Input: part model. Units: mm. Frame: model coordinates. A direction names the side the tool comes from. Give positions to 0.01 mm unless a question says otherwise; leave off trailing zeros. Loops run counter-clockwise (first coordinate to the right, second up) from the corner with the lowest first, then second, coordinate; pieces in that order, holes last. Notation, with made-up numbers: (-30, 35) -> (1, 35) arc R10 cw to (1, 39) -> close; hole circle Ø5 at (38.5, 81.5). An arc over 180 degrees is marked (long way). Answer as a JSON object with one key per item and string values. Group by question number.
Autodesk Inventor part; units mm, degrees
ref_plane "YZ Plane" through (0, 0, 0) normal (1, 0, 0) x (0, 1, 0)
ref_plane "XZ Plane" through (0, 0, 0) normal (0, 1, 0) x (-1, 0, 0)
ref_plane "XY Plane" through (0, 0, 0) normal (0, 0, 1) x (1, 0, 0)
sketch "Sketch2" plane through (0, 0, 0) normal (0, 0, 1) x (1, 0, 0)
  line L0 (0, 12.7) -> (3.6703, 12.7)
  line L1 (0, 12.7) -> (-3.6703, 12.7)
  line L2 (0, 0) -> (3.6703, 0)
  line L3 (0, 0) -> (-3.6703, 0)
  line L4 (-3.6703, 0) -> (-7.3406, 6.35)
  line L5 (-7.3406, 6.35) -> (-3.6703, 12.7)
  line L6 (3.6703, 12.7) -> (7.3406, 6.35)
  line L7 (7.3406, 6.35) -> (3.6703, 0)
  line L8 (0, 0) -> (0, 6.35)
  circle A0 centre (0, 6.35) radius 8.255
  dimension "d11" = 6.35
  dimension "d12" = 16.51
extrude "Extrusion2" add sketch "Sketch2" along normal blind 6.223
sketch "Sketch3" plane through (0, 6.35, 6.223) normal (0, 0, 1) x (1, 0, 0)
  line L0 (-3.6703, -6.35) -> (-7.3406, 0)
  line L1 (-7.3406, 0) -> (-3.6703, 6.35)
  line L2 (-3.6703, 6.35) -> (3.6703, 6.35)
  line L3 (3.6703, 6.35) -> (7.3406, 0)
  line L4 (7.3406, 0) -> (3.6703, -6.35)
  line L5 (3.6703, -6.35) -> (-3.6703, -6.35)
  circle A0 centre (0, 0) radius 8.255
  point P0 (0, -6.35)
extrude "Extrusion3" add sketch "Sketch3" along normal blind 3.302
sketch "Sketch4" plane through (0, 6.35, 9.525) normal (0, 0, 1) x (1, 0, 0)
  line L0 (-7.3406, 0) -> (-3.6703, 6.35)
  line L1 (-3.6703, 6.35) -> (3.6703, 6.35)
  line L2 (3.6703, 6.35) -> (7.3406, 0)
  line L3 (7.3406, 0) -> (3.6703, -6.35)
  line L4 (3.6703, -6.35) -> (-3.6703, -6.35)
  line L5 (-3.6703, -6.35) -> (-7.3406, 0)
  circle A0 centre (0, 0) radius 8.255
  point P0 (0, -6.35)
extrude "Extrusion4" add sketch "Sketch4" along normal blind 6.5786
sketch "Sketch5" plane through (0, 6.35, 16.1036) normal (0, 0, 1) x (1, 0, 0)
  line L0 (-16.3467, 15.7745) -> (15.1254, 15.7745)
  line L1 (15.1254, 15.7745) -> (15.1254, -12.8793)
  line L2 (15.1254, -12.8793) -> (-16.3467, -12.8793)
  line L3 (-16.3467, -12.8793) -> (-16.3467, 15.7745)
  point P0 (0, -6.35)
extrude "Extrusion5" cut sketch "Sketch5" against normal blind 6.5786
sketch "Sketch8" plane through (0, 6.35, 9.525) normal (0, 0, 1) x (1, 0, 0)
  line L0 (-7.3406, 0) -> (-3.6703, -6.35)
  line L1 (-3.6703, 6.35) -> (-7.3406, 0)
  line L2 (3.6703, 6.35) -> (-3.6703, 6.35)
  line L3 (7.3406, 0) -> (3.6703, 6.35)
  line L4 (3.6703, -6.35) -> (7.3406, 0)
  line L5 (-3.6703, -6.35) -> (3.6703, -6.35)
  circle A0 centre (0, 0) radius 8.255
  point P0 (0, -6.35)
extrude "Extrusion7" add sketch "Sketch8" along normal blind 15.875
sketch "Sketch9" plane through (0, 6.35, 25.4) normal (0, 0, 1) x (1, 0, 0)
  line L0 (-7.3406, 0) -> (-3.6703, 6.35)
  line L1 (-3.6703, 6.35) -> (3.6703, 6.35)
  line L2 (3.6703, 6.35) -> (7.3406, 0)
  line L3 (7.3406, 0) -> (3.6703, -6.35)
  line L4 (3.6703, -6.35) -> (-3.6703, -6.35)
  line L5 (-3.6703, -6.35) -> (-7.3406, 0)
  circle A0 centre (0, 0) radius 8.255
  point P0 (0, -6.35)
extrude "Extrusion8" cut sketch "Sketch9" against normal blind 21.7424
sketch "Sketch10" plane through (0, 6.35, 3.6576) normal (0, 0, 1) x (1, 0, 0)
  line L0 (-7.3406, 0) -> (-3.6703, -6.35)
  line L1 (-3.6703, 6.35) -> (-7.3406, 0)
  line L2 (3.6703, 6.35) -> (-3.6703, 6.35)
  line L3 (7.3406, 0) -> (3.6703, 6.35)
  line L4 (3.6703, -6.35) -> (7.3406, 0)
  line L5 (-3.6703, -6.35) -> (3.6703, -6.35)
  circle A0 centre (0, 0) radius 8.255
  point P0 (0, -6.35)
extrude "Extrusion9" add sketch "Sketch10" along normal blind 9.1948
sketch "Sketch11" plane through (0, 6.35, 12.8524) normal (0, 0, 1) x (1, 0, 0)
  line L0 (-10.961, 11.9872) -> (13.8218, 11.9872)
  line L1 (13.8218, 11.9872) -> (13.8218, -11.21)
  line L2 (13.8218, -11.21) -> (-10.961, -11.21)
  line L3 (-10.961, -11.21) -> (-10.961, 11.9872)
  point P0 (0, -6.35)
extrude "Extrusion10" cut sketch "Sketch11" against normal blind 10.16
properties part number ".106Spacer"
Q1. Ray query, probe 1 along Y at (x, z) = (0, 0.95) (3 decimals); probe 2 along Y at (x, z) = (-7.25, 1.3); probe 3 along X at (y, z) = (11.25, 2.35). Return the intervals inside material, ascending.
Q2. Pull-direction query (X, two-part tool) for faces 3 (the face through (-5, 2, 0)), 4 (the face through (-1.79, 14.41, 1.33)), 5 (the face through (5.48, 3.13, 1.33)), 6 (the face through (5.53, 9.48, 1.33)); classes: +X half, -X half, draft (parallel to the pull), parting line (faces both ways), or undercut.
Q3. Section C-C on y = 8. Return the cut outline in (x, z).
Q4. Set-up query: faces 1 (the face through (0, 12.7, 1)), 2 (the face through (-5, 2, 2.692)). Return all of +Z, -Z, +X, -X, +Y, -Y with unobstructed straight access to the full face (end or side cutting, diameter ignored); none if empty.
Q5. Pin query (flat end, axial travel): pin 1 Ø0.8 at (x, z) = (-0.5, 1) entering from -Y; pin 2 Ø1 at (y, z) = (1, 2) entering from +X. Return the tip coordinate at first contact, or that it passes through.
Q6. Section B-B on z = 1.75. Return the cut outline in (x, y) (3 decimals), then the cut area to 3 significant figures.
Q7. Section A-A on x = 0. Return the cut outline in (y, z) (3 decimals).
Numbers:
{
 "1": {"probe 1": "y = -1.905 to 0, 12.7 to 14.605", "probe 2": "y = 2.4 to 6.19, 6.51 to 10.3", "probe 3": "x = -6.64 to -4.51, 4.51 to 6.64"},
 "2": {"face 3": "draft", "face 4": "parting line", "face 5": "undercut", "face 6": "undercut"},
 "3": {"outline": "(-8.09, 0) -> (-6.39, 0) -> (-6.39, 2.69) -> (-8.09, 2.69) -> close; (6.39, 0) -> (8.09, 0) -> (8.09, 2.69) -> (6.39, 2.69) -> close"},
 "4": {"face 1": "+Z, -Z", "face 2": "+Z, +X, -X, +Y, -Y"},
 "5": {"pin 1": "stops at y = -1.9", "pin 2": "stops at x = 6.68"},
 "6": {"outline": "circle Ø16.51 at (0, 6.35); hole (-7.341, 6.35) -> (-3.67, 0) -> (3.67, 0) -> (7.341, 6.35) -> (3.67, 12.7) -> (-3.67, 12.7) -> close", "area": "74.2 mm²"},
 "7": {"outline": "(-1.905, 0) -> (0, 0) -> (0, 2.692) -> (-1.905, 2.692) -> close; (12.7, 0) -> (14.605, 0) -> (14.605, 2.692) -> (12.7, 2.692) -> close"}
}
